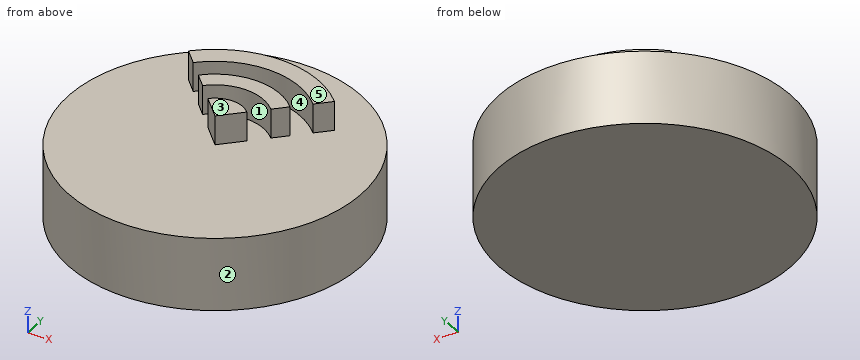
from build123d import *

# Parameters (mm, degrees)
F0_R     = 5
F1_DEPTH = 2.5
F3_DEPTH = 1


with BuildPart() as f1:
    # F0 (on Top) → F1 (new body)
    with BuildSketch(Plane.XY):
        Circle(F0_R)
    extrude(amount=F1_DEPTH)

    # F2 (on face) → F3 (join)
    with BuildSketch(Plane.XY.offset(2.5)):
        with BuildLine():
            Line((2.062848, 2.062848), (2.513184, 2.513184))
            ThreePointArc((2.513184, 2.513184), (0, 3.55418), (-2.513184, 2.513184))
            Line((-2.513184, 2.513184), (-2.062848, 2.062848))
            ThreePointArc((-2.062848, 2.062848), (0, 2.917307), (2.062848, 2.062848))
        make_face()
        with BuildLine():
            Line((1.173422, 1.173422), (1.577984, 1.577984))
            ThreePointArc((1.577984, 1.577984), (0, 2.231606), (-1.577984, 1.577984))
            Line((-1.577984, 1.577984), (-1.173422, 1.173422))
            ThreePointArc((-1.173422, 1.173422), (0, 1.659469), (1.173422, 1.173422))
        make_face()
        with BuildLine():
            Line((0, 0), (0.670121, 0.670121))
            ThreePointArc((0.670121, 0.670121), (0, 0.947694), (-0.670121, 0.670121))
            Line((-0.670121, 0.670121), (0, 0))
        make_face()
    extrude(amount=F3_DEPTH)


solid = f1.part
The model under review builds one solid part; all positions refer to its coordinate system, in mm. Face numbers are marked on the shaded views. A direction names the side the tool comes from. Give positions to 0.01 mm unless a question says otherwise; leave off trailing zeros. Loops run counter-clockwise (first coordinate to the right, second up) from the corner with the lowest first, then second, coordinate; pieces in that order, holes last. Notation, with made-up numbers: (89.5, 64.5) -> (128.5, 64.5) arc R9 cw to (128.5, 71.5) -> close; hole circle Ø8 at (44, 50). An arc over 180 degrees is marked (long way). Write each question's results on one line, items separated by ' | '.
1) Take a section at D-D, the plane y = -3.25. Give the boundary of the cut face in (x, z), plus the area to 3 significant figures.
Conclusion:
outline: (-3.8, 0) -> (3.8, 0) -> (3.8, 2.5) -> (-3.8, 2.5) -> close | area: 19.0 mm^2
2) Take a section at C-C, the plane z = 0.95. Give the boundary of the cut face in (x, y).
Conclusion:
outline: circle Ø10 at (0, 0)
3) Draft analysis for pull direction X (two halves, no side actions). For the marked faces 1, 2 and 3, state which applies: pulls with the +X half, pulls with the -X half, needs draft (parallel to the pull), parting line crosses it, or undercut.
Conclusion:
face 1: undercut | face 2: parting line crosses it | face 3: needs draft
4) Insertion check: pin 1 Ø2 at (x, y) = (2.5, 0) entering from +Z; pin 2 Ø2 at (y, z) = (-3, 1.5) entering from +X; pin 3 Ø2 at (x, z) = (-2, 1) entering from +Y; pin 4 Ø3 at (x, y) = (-2, 1.5) entering from +Z. Each pin has a flat end and moves straight along its axis. Give the tip position at first contact, or say it passes through.
Conclusion:
pin 1: stops at z = 2.5 | pin 2: stops at x = 4.58 | pin 3: stops at y = 4.9 | pin 4: stops at z = 3.5
5) For line 1 along Z through (x, y) = (4, -1.25); line 2 along X through (y, z) = (4, 0.35); line 3 along X through (y, z) = (3.5, 1), list the stretches that pass through material, from the lowest coordinate up. Write a range as from..to.
Conclusion:
line 1: z = 0..2.5 | line 2: x = -3..3 | line 3: x = -3.57..3.57
6) Tool access review of the marked faces 4 and 5: name each direction out of +Z, -Z, +X, -X, +Y, -Y from which nothing blocks a thin tool from reaching the whole face with its end or side.
Conclusion:
face 4: +Z | face 5: +Z, +X, -X, +Y, -Y
7) Take a section at B-B, the plane x = 3. Give the boundary of the cut face in (y, z).
Conclusion:
outline: (-4, 0) -> (4, 0) -> (4, 2.5) -> (-4, 2.5) -> close
8) Take a section at A-A, the plane z = 3.1. Give the boundary of the cut face in (x, y).
Conclusion:
outline: (-2.51, 2.51) -> (-2.06, 2.06) arc R2.92 cw to (2.06, 2.06) -> (2.51, 2.51) arc R3.55 ccw to start; (-1.58, 1.58) -> (-1.17, 1.17) arc R1.66 cw to (1.17, 1.17) -> (1.58, 1.58) arc R2.23 ccw to start; (-0.67, 0.67) -> (0, 0) -> (0.67, 0.67) arc R0.95 ccw to start
